Could you check a few things on this model? Use its own coordinates, in mm. Face numbers are marked on the shaded views. Give positions to 0.01 mm unless a question says otherwise; leave off trailing zeros. Loops run counter-clockwise (first coordinate to the right, second up) from the corner with the lowest first, then second, coordinate; pieces in that order, holes last. Notation, with made-up numbers: (19.25, 18) - (60.25, 18) arc R27 cw to (60.25, 49) - close; hole circle Ø7 at (2.5, 79). An arc over 180 degrees is marked (long way). One line per item, written item: value. Start each with the question number.
Q1. If we mould it in two halves opening along Z, with no side actions, what happens to the marked faces 1, 2 and 3? For each: released by +Z, released by -Z, zero draft, split by the parting line, or undercut.
Q2. I want a section at C-C (x = 11.5). Please give me the cut outline in (y, z), then the cut area to 3 significant figures.
Q3. I want a section at A-A (x = 4). Please give me the cut outline in (y, z).
Q4. I'm going to push flat-ended pins straight in: P1, Ø5, axis at x = 15.5, y = 1.5, coming from the +Z side; P2, Ø3, axis at y = 2.5, z = -2, coming from the +X side; P3, Ø6, axis at x = 25, z = 7.5, coming from the +Y side. Where does each tip first touch, or does it pass through?
Q5. I want a section at B-B (x = 16.5). Please give me the cut outline in (y, z) (3 decimals).
Q6. If I drill on line 1 (Y direction, x = 18, z = 0) (3 decimals); line 2 (Y direction, x = 17, z = -1.75); line 3 (X direction, y = 2.75, z = -2.75), over which ranges is the centre line in solid material (lowest first)? Write a range as from..to.
```python
from build123d import *

# Parameters (mm, degrees)
F2_R     = 1.7526
F3_DEPTH = 5.08
F4_R     = 0.3048


with BuildPart() as f1:
    # F0 (on Front) → F1 (revolve)
    with BuildSketch(Plane.XZ):
        Polygon((0, 12.6238), (0, 0), (13.843, 0), (13.843, 3.175), (24.003, 3.175), (24.003, 4.8133), (24.5618, 4.8133), (24.5618, 12.6238), (23.4442, 12.6238), align=None)
        with BuildLine():
            ThreePointArc((24.5618, 12.6238), (24.003, 12.636162), (23.4442, 12.6238))
            Line((23.4442, 12.6238), (24.5618, 12.6238))
        make_face()
        with BuildLine():
            ThreePointArc((33.8836, 7.876949), (29.73697, 11.260292), (24.5618, 12.6238))
            Line((24.5618, 12.6238), (24.5618, 4.8133))
            Line((24.5618, 4.8133), (33.8836, 4.8133))
            Line((33.8836, 4.8133), (33.8836, 7.876949))
        make_face()
    revolve(axis=Axis((6.9215, 0, 0), (-1, 0, 0)))

    # F2 (on face) → F3 (cut)
    with BuildSketch(Plane(origin=(0, 0, 0), x_dir=(0, -1, 0), z_dir=(-1, 0, 0))):
        with Locations((0, 6.35)):
            Circle(F2_R)
        with Locations((-6.35, 0)):
            Circle(F2_R)
        with Locations((0, -6.35)):
            Circle(F2_R)
        with Locations((6.35, 0)):
            Circle(F2_R)
    extrude(amount=-F3_DEPTH, mode=Mode.SUBTRACT)

    # F4
    f4_edges = [f1.edges().sort_by_distance(p)[0] for p in [
        (0, 0, -12.6238),
    ]]
    fillet(f4_edges, radius=F4_R)


solid = f1.part
```
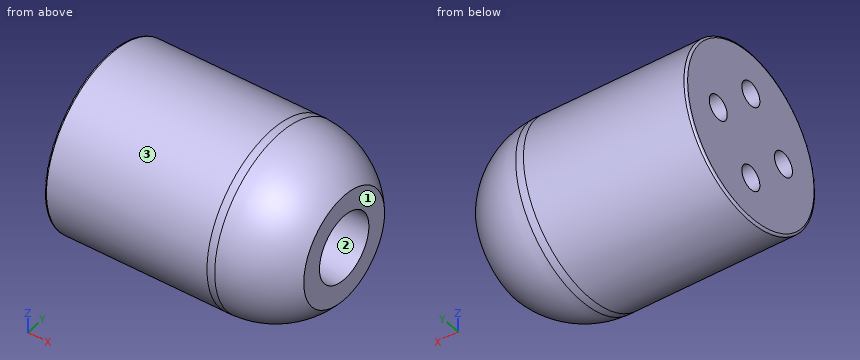
Worked answers:
1. face 1: zero draft
1. face 2: undercut
1. face 3: split by the parting line
2. outline: circle Ø25.25 at (0, 0)
2. area: 501 mm²
3. outline: circle Ø25.25 at (0, 0); hole circle Ø3.51 at (-6.35, 0); hole circle Ø3.51 at (0, -6.35); hole circle Ø3.51 at (0, 6.35); hole circle Ø3.51 at (6.35, 0)
4. P1: stops at z = 12.62
4. P2: stops at x = 24
4. P3: stops at y = 11.78
5. outline: circle Ø25.248 at (0, 0); hole circle Ø6.35 at (0, 0)
6. line 1: y = -12.624..-3.175, 3.175..12.624
6. line 2: y = -12.5..-2.65, 2.65..12.5
6. line 3: x = 0..24
